Here's the drawing with two shaded views (mm, measured from the low corner). I have some questions. A direction names the side the tool comes from. Give positions to 0.01 mm unless a question says otherwise; leave off trailing zeros. Write each loop counter-clockwise with the first axis right and the second up, starting at its lowest first coordinate (ties: lowest second). Pieces come first, ordered by that corner, then holes. Notation, with made-up numbers: M 39,-27 L 43,-27 A28 cw 43,-7 Z; hole C 79,81 d9. An arc over 180 degrees is marked long. Use one line per item in the form item = value.
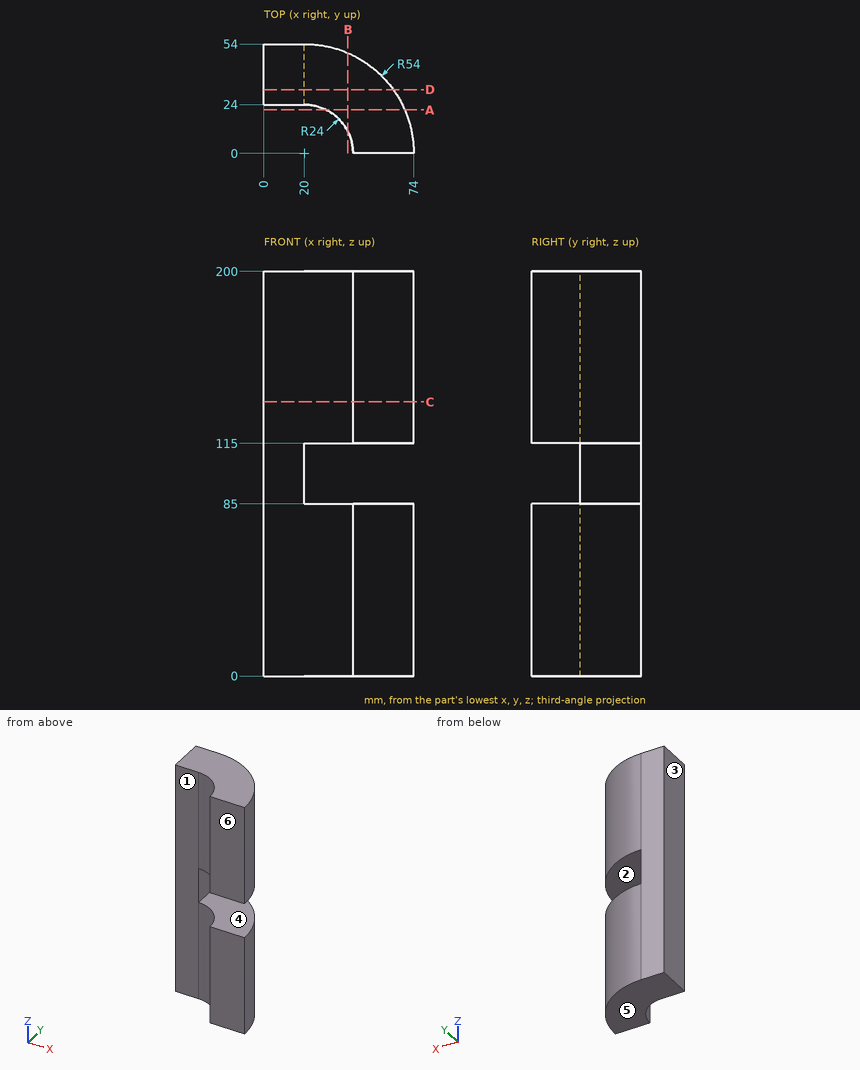
1) If I drill on L1, parallel to Z at x = 46, y = 6; L2, parallel to Y at x = 19.5, z = 19.5; L3, parallel to X at y = 33, z = 87, over which ranges is the centre line in solid material (lowest first)?
Checked values:
L1 = 0 to 85, 115 to 200
L2 = 24 to 54
L3 = 0 to 20
2) For pin 1 Ø12 at (x, y) = (58.5, 34.5) entering from -Z; pin 2 Ø1.5 at (x, z) = (11.5, 61.5) entering from -Y; pin 3 Ø1.5 at (x, z) = (36, 138) entering from -Y; pin 4 Ø6 at (x, z) = (30, 72) entering from +Y, each with a flat end and sliding along its axis, tell me the tip position at first contact or that it passes through.
Checked values:
pin_1 = 0
pin_2 = 24
pin_3 = 17.19
pin_4 = 53.54
3) I want a section at A-A, the plane y = 21.5. Please give me the cut outline in (x, z), plus the area to 3 significant figures.
Checked values:
outline = M 30.67,0 L 69.54,0 L 69.54,85 L 30.67,85 Z; M 30.67,115 L 69.54,115 L 69.54,200 L 30.67,200 Z
area = 6,610 mm2
4) I want a section at D-D, the plane y = 31.5. Please give me the cut outline in (x, z).
Checked values:
outline = M 0,0 L 63.86,0 L 63.86,85 L 20,85 L 20,115 L 63.86,115 L 63.86,200 L 0,200 Z
5) I want a section at B-B, the plane x = 41.5. Please give me the cut outline in (y, z), plus the area to 3 significant figures.
Checked values:
outline = M 10.67,0 L 49.54,0 L 49.54,85 L 10.67,85 Z; M 10.67,115 L 49.54,115 L 49.54,200 L 10.67,200 Z
area = 6,610 mm2
6) I want a section at C-C, the plane z = 135.5. Please give me the cut outline in (x, y), plus the area to 3 significant figures.
Checked values:
outline = M 0,24 L 20,24 A24 cw 44,0 L 74,0 A54 ccw 20,54 L 0,54 Z
area = 2,440 mm2
7) For the marked faces 1, 2 and 3, which set-ups out of +Z, -Z, +X, -X, +Y, -Y let a thin tool reach every point of the face, with its end or its side?
Checked values:
face_1 = +Z, -Z, -X, -Y
face_2 = +X, +Y, -Y
face_3 = +Z, -Z, -X, +Y, -Y
8) Thinking about a two-plate mould opening in Z: for the marked faces 4, 5 and 6, which applies, released by +Z, released by -Z, zero draft, split by the parting line, or undercut?
Checked values:
face_4 = undercut
face_5 = released by -Z
face_6 = zero draft
